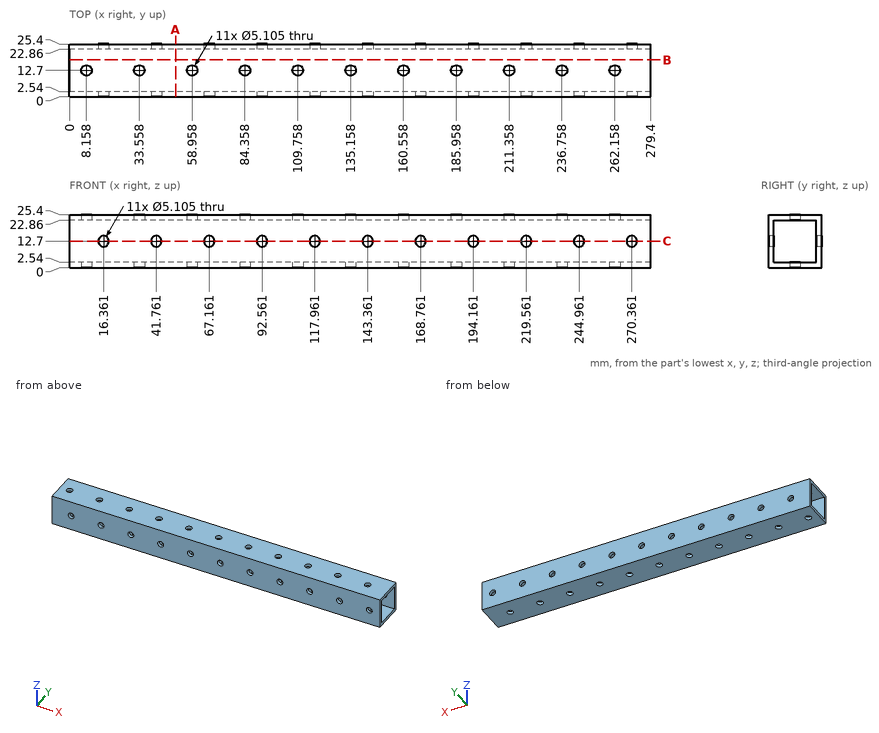
Here's the drawing with two shaded views (mm, measured from the low corner). I have some questions. Coordinates: 2 decimals unless noted, no trailing zeros. Write each loop counter-clockwise with the first axis right and the second up, starting at its lowest first coordinate (ties: lowest second). Pieces come first, ordered by that corner, then holes.
Item 1: If I drill on line 1 (Z direction, x = 196, y = 6.75); line 2 (Z direction, x = 69, y = 23), over which ranges is the centre line in solid material (lowest first)?
Item 2: I want a section at B-B on y = 17.75. Write out the boundary of the cut face in (x, z).
Item 3: I want a section at C-C on z = 12.7. Count the separate pieces of the cut face and the enclosed holes in it, and give its area (3 significant figures).
Item 4: I want a section at A-A on x = 51. Write out the boundary of the cut face in (y, z).
Item 5: Will this pin go through, and if not, where does the flat tip stop? pin 1 (4.5 mm diameter, centred on x = 219.56, z = 12.7, fed in from -Y).
Findings below:
1. line 1: z = 0 to 2.54, 22.86 to 25.4
1. line 2: z = 0 to 10.93, 14.47 to 25.4
2. outline: (0, 0) - (279.4, 0) - (279.4, 2.54) - (0, 2.54) - close; (0, 22.86) - (279.4, 22.86) - (279.4, 25.4) - (0, 25.4) - close
3. separate pieces: 24
3. enclosed holes: 0
3. area: 1,130 mm2
4. outline: (0, 0) - (25.4, 0) - (25.4, 25.4) - (0, 25.4) - close; hole (2.54, 2.54) - (22.86, 2.54) - (22.86, 22.86) - (2.54, 22.86) - close
5. pin 1: passes through
